```python
from build123d import *

# Parameters (mm, degrees)
SCHIZZO1_R                    = 9.9
ESTRUSIONE_ESTRUSIONE1_DEPTH  = 29.8
TAGLIO_ESTRUSIONE1_DEPTH      = 33.925066439
TAGLIO_ESTRUSIONE1_DEPTH_BACK = 33.925066439
SCHIZZO3_R                    = 4.15
SCHIZZO5_R                    = 9.9
ESTRUSIONE_ESTRUSIONE2_DEPTH  = 8
SCHIZZO6_R                    = 3.1
TAGLIO_ESTRUSIONE3_DEPTH      = 2
SCHIZZO7_R                    = 2.9
TAGLIO_ESTRUSIONE4_DEPTH      = 1.85
SCHIZZO8_R                    = 1.25
TAGLIO_ESTRUSIONE5_DEPTH      = 10


with BuildPart() as part:
    # Schizzo1 → Estrusione-Estrusione1 (new body)
    with BuildSketch(Plane.XY):
        Circle(SCHIZZO1_R)
    extrude(amount=ESTRUSIONE_ESTRUSIONE1_DEPTH)

    # Schizzo3 → Taglio-Estrusione1 (cut, two sides: drawn at the far end of the back side and taken through both)
    with BuildSketch(Plane(origin=(0, 0, 0), x_dir=(0, 0, -1), z_dir=(1, 0, 0)).offset(-TAGLIO_ESTRUSIONE1_DEPTH_BACK)):
        with Locations((-16.9, 0)):
            Circle(SCHIZZO3_R)
    extrude(amount=TAGLIO_ESTRUSIONE1_DEPTH + TAGLIO_ESTRUSIONE1_DEPTH_BACK, mode=Mode.SUBTRACT)

    # Schizzo5 → Estrusione-Estrusione2 (add)
    with BuildSketch(Plane.XY.offset(29.8)):
        Circle(SCHIZZO5_R)
    extrude(amount=ESTRUSIONE_ESTRUSIONE2_DEPTH)

    # Schizzo6 → Taglio-Estrusione3 (cut)
    with BuildSketch(Plane.XY.offset(37.8)):
        Circle(SCHIZZO6_R)
    extrude(amount=-TAGLIO_ESTRUSIONE3_DEPTH, mode=Mode.SUBTRACT)

    # Schizzo7 → Taglio-Estrusione4 (cut)
    with BuildSketch(Plane.XY.offset(35.8)):
        Circle(SCHIZZO7_R)
    extrude(amount=-TAGLIO_ESTRUSIONE4_DEPTH, mode=Mode.SUBTRACT)

    # Schizzo8 → Taglio-Estrusione5 (cut)
    with BuildSketch(Plane.XY.offset(33.95)):
        Circle(SCHIZZO8_R)
    extrude(amount=-TAGLIO_ESTRUSIONE5_DEPTH, mode=Mode.SUBTRACT)


solid = part.part
```
Work out the finished part from the listing and answer in its coordinate system (mm). A direction names the side the tool comes from. Give positions to 0.01 mm unless a question says otherwise; leave off trailing zeros. Order: outer loops, then holes, each group sorted by start corner. A loop starts at its lowest first (then second) coordinate and runs counter-clockwise, first axis right, second up. Notation, with made-up numbers: (-20.5, 14) - (37.5, 14) arc R11 cw to (37.5, 32) - close; hole circle Ø7 at (-29.5, 68). An arc over 180 degrees is marked (long way). One line per item, written item: value. Start each with the question number.
1. Section A-A, the plane x = 0 is taken. Write down the section's boundary in (y, z), then the cut area to 3 significant figures.
2. Consider line 1 (Z direction, x = 4.5, y = 0); line 2 (Y direction, x = 0, z = 34.8); line 3 (Y direction, x = 0, z = 27.25). Determine where each line is inside the solid, lowest interval first.
3. Which of the six approach directions +Z, -Z, +X, -X, +Y, -Y give full straight-line access (tool end or side, diameter ignored) to faces 1 (the face through (-0.142, 1.247, 12.942)), 2 (the face through (1.43, -2.75, 36.81))?
4. Each of these flat-tipped pins is pushed along its axis until it touches: pin 1 Ø10 at (x, z) = (-8, 9.5) entering from -Y; pin 2 Ø3.5 at (x, y) = (0, 0) entering from +Z; pin 3 Ø10 at (y, z) = (7.5, 13) entering from -X; pin 4 Ø7 at (x, y) = (1.5, 1) entering from +Z. Where does it stop, or does it pass through?
5. Section B-B, the plane y = 0 is taken. Write down the section's boundary in (x, z), then the cut area to 3 significant figures.
6. Section C-C, the plane z = 27 is taken. Write down the section's boundary in (x, y).
7. Section D-D, the plane z = 22.5 is taken. Write down the section's boundary in (x, y).
8. For a pull along X with two mould halves and no side action, classify faces 3 (the face through (-2.146, -9.665, 18.635)), 4 (the face through (0, 0, 23.95)), 5 (the face through (0, 0, 0)) as released by +X, released by -X, zero draft, split by the parting line, or undercut.
Filled sheet:
1. outline: (-9.9, 0) - (9.9, 0) - (9.9, 37.8) - (3.1, 37.8) - (3.1, 35.8) - (2.9, 35.8) - (2.9, 33.95) - (1.25, 33.95) - (1.25, 23.95) - (-1.25, 23.95) - (-1.25, 33.95) - (-2.9, 33.95) - (-2.9, 35.8) - (-3.1, 35.8) - (-3.1, 37.8) - (-9.9, 37.8) - close; hole circle Ø8.3 at (0, 16.9)
1. area: 646 mm²
2. line 1: 0 to 12.75, 21.05 to 37.8
2. line 2: -9.9 to -2.9, 2.9 to 9.9
2. line 3: -9.9 to -1.25, 1.25 to 9.9
3. face 1: +X, -X
3. face 2: +Z
4. pin 1: y = -9.43
4. pin 2: z = 33.95
4. pin 3: x = -9.58
4. pin 4: z = 37.8
5. outline: (-9.9, 0) - (9.9, 0) - (9.9, 12.75) - (-9.9, 12.75) - close; (-9.9, 21.05) - (9.9, 21.05) - (9.9, 37.8) - (3.1, 37.8) - (3.1, 35.8) - (2.9, 35.8) - (2.9, 33.95) - (1.25, 33.95) - (1.25, 23.95) - (-1.25, 23.95) - (-1.25, 33.95) - (-2.9, 33.95) - (-2.9, 35.8) - (-3.1, 35.8) - (-3.1, 37.8) - (-9.9, 37.8) - close
5. area: 536 mm²
6. outline: circle Ø19.8 at (0, 0); hole circle Ø2.5 at (0, 0)
7. outline: circle Ø19.8 at (0, 0)
8. face 3: split by the parting line
8. face 4: undercut
8. face 5: zero draft
